Check sheet for the modelled part. Datum: model origin and axes. Units: mm. Face numbers are marked on the shaded views. A direction names the side the tool comes from. Coordinates: 2 decimals unless noted, no trailing zeros. Loops run counter-clockwise (first coordinate to the right, second up) from the corner with the lowest first, then second, coordinate; pieces in that order, holes last. Notation, with made-up numbers: M 39,19.25 L 92,19.25 A17 cw 92,48.25 Z; hole C -36,35 d1. An arc over 180 degrees is marked long. Use CSV: the item, a comma, the result in double quotes. Start each with the question number.
(1) Set-up check for the marked faces 1 and 2: record each of +Z, -Z, +X, -X, +Y, -Y from which the full face is reachable in a straight line by a thin tool's end or side.
(2) Section check B-B on z = 27. Record the cut outline in (x, y), and give its area (3 significant figures).
(3) Section check C-C on z = 15.5. Record the cut outline in (x, y), and give its area (3 significant figures).
(4) Scan lines: line 1 (Y direction, x = 0, z = 1); line 2 (Y direction, x = -9, z = 9); line 3 (Z direction, x = 24, y = -39). Record each from-to range of solid material in increasing order.
(5) Section check A-A on x = 0. Record the cut outline in (y, z), and give its area (3 significant figures).
(6) Go/stop test with flat-tipped pins: pin 1 Ø1.5 at (y, z) = (-7, 14.5) entering from -X; pin 2 Ø5 at (y, z) = (-5, -2.5) entering from -X; pin 3 Ø2 at (x, z) = (1, -3.5) entering from +Y. Record where each tip stops, or that it passes through.
Autodesk Inventor part; units mm, degrees
ref_plane "YZ Plane" through (0, 0, 0) normal (1, 0, 0) x (0, 1, 0)
ref_plane "XZ Plane" through (0, 0, 0) normal (0, 1, 0) x (-1, 0, 0)
ref_plane "XY Plane" through (0, 0, 0) normal (0, 0, 1) x (1, 0, 0)
sketch "Szkic7" plane through (0, 0, 0) normal (0, 0, 1) x (1, 0, 0)
  circle A0 centre (0, 0) radius 43.942
  dimension "d35" = 87.884
extrude "Wyciągnięcie proste2" add sketch "Szkic7" along normal mid plane 39.825
chamfer "Faza2" distance 1 angle 45 1 edges at (-43.942, 0, 19.9125)
sketch "Szkic9" plane through (0, 0, 19.9125) normal (0, 0, 1) x (1, 0, 0)
  circle A0 centre (0, 0) radius 42.942
extrude "Wyciągnięcie proste3" add sketch "Szkic9" along normal blind 3.375
sketch "Szkic10" plane through (0, 0, 23.2875) normal (0, 0, 1) x (1, 0, 0)
  line L0 (-27.1355, 47) -> (27.1355, 47)
  line L1 (27.1355, 47) -> (54.2709, 0)
  line L2 (54.2709, 0) -> (27.1355, -47)
  line L3 (27.1355, -47) -> (-27.1355, -47)
  line L4 (-27.1355, -47) -> (-54.2709, 0)
  line L5 (-54.2709, 0) -> (-27.1355, 47)
  line L6 (0, 61.5188) -> (0, -61.5188) construction
  line L7 (-61.5188, 0) -> (61.5188, 0) construction
  point P0 (0, 0)
  point P1 (0, 0)
  point P2 (0, 47)
  dimension "d44" = 94
extrude "Wyciągnięcie proste4" add sketch "Szkic10" along normal blind 10.8
sketch "Szkic12" plane through (0, 0, 0) normal (0, 1, 0) x (-1, 0, 0)
  line L0 (0, -2.1463) -> (0, 12.8775) construction
  line L1 (-27.1355, 23.2875) -> (-27.1355, 34.0875) construction
  line L2 (-54.2709, 34.0875) -> (-27.1355, 34.0875) construction
  line L3 (-54.2709, 23.2875) -> (-54.2709, 34.0875)
  line L4 (-54.2709, 32.4084) -> (-48.0043, 34.0875)
  line L5 (-54.2709, 34.0875) -> (-27.1355, 34.0875)
  line L6 (-54.2709, 23.2875) -> (-27.1355, 23.2875)
  point P0 (0, 0)
  dimension "d50" = 15
  dimension "d51" = 6.2667
revolve "Obrót2" cut sketch "Szkic12" angle 360 about axis through (0, 0, -10) along (0, 0, 1)
thread "Gwint3"
chamfer "Faza3" distance 1 angle 45 1 edges at (-43.942, 0, -19.9125)
equation "\"d35\" = OD"
equation "\"d36\" = 0.7375 * L"
equation "\"d42\" = 0.0625 * L"
equation "\"d44\" = SW"
equation "\"d45\" = 0.2 * L"
equation "\"d51\" = 0.0666667 * SW"
equation "\"SzerokośćGięciaPodcięcia\" = Grubość"
equation "\"RozmiarPodcięciaNarożnika\" = 4 * Grubość"
equation "\"PromieńPrzejścia\" = PromieńGięcia"
equation "\"Rozmiar_promienia_Jacobiego\" = PromieńGięcia"
equation "\"Wielk_odstępu\" = Grubość"
equation "\"d2\" = PromieńGięcia"
equation "\"d23\" = PromieńGięcia"
equation "\"OD\" = 87.884"
equation "\"SW\" = 94"
equation "\"L\" = 54"
properties part number "Korek sześciokątny BSP 3'' L=54" material "304"
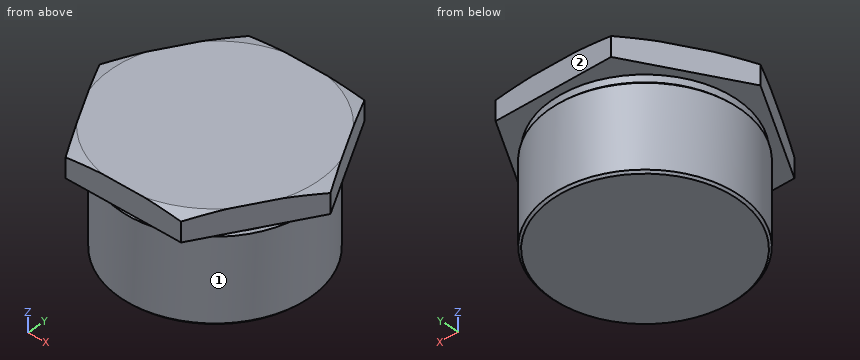
Outcome:
1,face 1,"-Z"
1,face 2,"+Z, -Z, +X, -X, +Y"
2,outline,"M -54.27,0 L -27.14,-47 L 27.14,-47 L 54.27,0 L 27.14,47 L -27.14,47 Z"
2,area,"7,650 mm²"
3,outline,"C 0,0 d87.88"
3,area,"6,070 mm²"
4,line 1,"y = -43.94 to 43.94"
4,line 2,"y = -43.01 to 43.01"
4,line 3,"z = 23.29 to 34.09"
5,outline,"M -47,23.29 L -42.94,23.29 L -42.94,19.91 L -43.94,18.91 L -43.94,-18.91 L -42.94,-19.91 L 42.94,-19.91 L 43.94,-18.91 L 43.94,18.91 L 42.94,19.91 L 42.94,23.29 L 47,23.29 L 47,34.09 L -47,34.09 Z"
5,area,"4,800 mm²"
6,pin 1,"stops at x = -43.5"
6,pin 2,"stops at x = -43.87"
6,pin 3,"stops at y = 43.94"
